```python
from build123d import *

# Parameters (mm, degrees)
SKETCH1_R                = 8
SKETCH1_R_2              = 2.5
BOSS_EXTRUDE1_DEPTH      = 2.5
BOSS_EXTRUDE1_DEPTH_BACK = 2.5
CUT_EXTRUDE1_START       = -2.5
SKETCH2_R                = 6.75
SKETCH2_R_2              = 3.75
CUT_EXTRUDE1_DEPTH       = 0.25
CUT_EXTRUDE2_START       = 2.5
SKETCH2_2_R              = 6.75
SKETCH2_2_R_2            = 3.75
CUT_EXTRUDE2_DEPTH       = 0.25
CHAMFER1_SIZE            = 0.1


with BuildPart() as part:
    # Sketch1 → Boss-Extrude1 (new body, two sides)
    with BuildSketch(Plane.XY) as boss_extrude1_sk:
        Circle(SKETCH1_R)
        Circle(SKETCH1_R_2, mode=Mode.SUBTRACT)
    extrude(amount=BOSS_EXTRUDE1_DEPTH)
    extrude(boss_extrude1_sk.sketch, amount=-BOSS_EXTRUDE1_DEPTH_BACK)

    # Sketch2 → Cut-Extrude1 (cut)
    with BuildSketch(Plane.XY.offset(CUT_EXTRUDE1_START)):
        Circle(SKETCH2_R)
        Circle(SKETCH2_R_2, mode=Mode.SUBTRACT)
    extrude(amount=CUT_EXTRUDE1_DEPTH, mode=Mode.SUBTRACT)

    # Sketch2_2 → Cut-Extrude2 (cut)
    with BuildSketch(Plane.XY.offset(CUT_EXTRUDE2_START)):
        Circle(SKETCH2_2_R)
        Circle(SKETCH2_2_R_2, mode=Mode.SUBTRACT)
    extrude(amount=-CUT_EXTRUDE2_DEPTH, mode=Mode.SUBTRACT)

    # Chamfer1
    chamfer1_edges = [part.edges().sort_by_distance(p)[0] for p in [
        (-3.75, 0, -2.5),
        (-6.75, 0, -2.5),
        (-6.75, 0, 2.5),
        (-3.75, 0, 2.5),
        (-8, 0, -2.5),
        (-2.5, 0, -2.5),
        (-8, 0, 2.5),
        (-2.5, 0, 2.5),
    ]]
    chamfer(chamfer1_edges, length=CHAMFER1_SIZE)


solid = part.part
```
Input: part model. Units: mm. Frame: model coordinates. A direction names the side the tool comes from. Give positions to 0.01 mm unless a question says otherwise; leave off trailing zeros. Order: outer loops, then holes, each group sorted by start corner. A loop starts at its lowest first (then second) coordinate and runs counter-clockwise, first axis right, second up. Notation, with made-up numbers: (-32, 71) - (5, 71) arc R29 cw to (5, 102) - close; hole circle Ø9 at (20, 29.25). An arc over 180 degrees is marked (long way). One line per item, written item: value.
1. Line query: probe 1 along Y at (x, z) = (0, -2.3); probe 2 along Z at (x, y) = (5.75, 1.5); probe 3 along Y at (x, z) = (0, -0.95). Output: solid intervals per line, ascending.
Determined:
probe 1: -8 to -6.75, -3.75 to -2.5, 2.5 to 3.75, 6.75 to 8
probe 2: -2.25 to 2.25
probe 3: -8 to -2.5, 2.5 to 8
2. Draft query along X for faces 1 (the face through (2, -2, -2.5)), 2 (the face through (3, -3, -2.25)), 3 (the face through (-1.73, -7.81, 0.03)). Return one class per face: released by +X, released by -X, zero draft, split by the parting line, or undercut.
Determined:
face 1: zero draft
face 2: undercut
face 3: split by the parting line
3. Reachability of faces 4 (the face through (-0.54, -2.44, -0.03)), 5 (the face through (3, -3, 2.25)) from +Z, -Z, +X, -X, +Y, -Y: full face, straight path, thin tool, end or side. Return the list, or none.
Determined:
face 4: +Z, -Z
face 5: +Z
4. Cut plane A-A, the plane z = -1.2. Output: boundary loops of the cut face in (x, y).
Determined:
outline: circle Ø16 at (0, 0); hole circle Ø5 at (0, 0)
5. Pin query (flat end, axial travel): pin 1 Ø3 at (x, y) = (0, 0) entering from -Z (3 decimals); pin 2 Ø2 at (x, z) = (6.5, 1.5) entering from +Y; pin 3 Ø3 at (y, z) = (-4.5, -1.5) entering from -X; pin 4 Ø3 at (x, z) = (-2, 1.5) entering from +Y. Return the tip coordinate at first contact, or that it passes through.
Determined:
pin 1: through
pin 2: y = 5.81
pin 3: x = -7.42
pin 4: y = 7.98
